```python
from build123d import *

# Parameters (mm, degrees)
F1_DEPTH        = 3.175
F2_R            = 6.35
F3_R            = 6.35
F5_DEPTH        = 34.7
F7_DEPTH        = 1.5875
F8_R            = 11.5
F9_DEPTH        = 215.1135
F11_D           = 4
F11_DEPTH       = 20
F11_START       = 1.5875
F11_CSINK_D     = 5
F11_CSINK_ANGLE = 90
F11_TIP         = 1.2017212381
F13_DEPTH       = 1.5875
F15_D           = 4
F15_DEPTH       = 20
F15_START       = 1.5875
F15_CSINK_D     = 5
F15_CSINK_ANGLE = 90
F15_TIP         = 1.2017212381
F17_D           = 4
F17_DEPTH       = 20
F17_TIP         = 1.2017212381
F20_D           = 4
F20_CSINK_D     = 8
F20_CSINK_ANGLE = 90


with BuildPart() as f1:
    # F0 (on Top) → F1 (new body)
    with BuildSketch(Plane.XY):
        Polygon((90.0875, 0), (0, 0), (0, -93.225), (216.7, -93.225), (216.7, -42.525), (126.6125, -42.525), (126.6125, 0), align=None)
    extrude(amount=F1_DEPTH)

    # F2
    f2_edges = [f1.edges().sort_by_distance(p)[0] for p in [
        (126.6125, -42.525, 1.5875),
    ]]
    fillet(f2_edges, radius=F2_R)

    # F3
    f3_edges = [f1.edges().sort_by_distance(p)[0] for p in [
        (216.7, -42.525, 1.5875),
        (216.7, -93.225, 1.5875),
        (0, -93.225, 1.5875),
        (0, 0, 1.5875),
    ]]
    fillet(f3_edges, radius=F3_R)

    # F4 (on face) → F5 (join)
    with BuildSketch(Plane.XY.offset(3.175)):
        with BuildLine():
            ThreePointArc((126.6125, -47.1735226281), (129.6754981272, -48.4422579939), (132.9625, -48.875))
            Line((132.9625, -48.875), (204, -48.875))
            ThreePointArc((204, -48.875), (208.4901280605, -50.7348719395), (210.35, -55.225))
            Line((210.35, -55.225), (210.35, -80.525))
            ThreePointArc((210.35, -80.525), (208.4901280605, -85.0151280605), (204, -86.875))
            Line((204, -86.875), (12.7, -86.875))
            ThreePointArc((12.7, -86.875), (8.2098719395, -85.0151280605), (6.35, -80.525))
            Line((6.35, -80.525), (6.35, -12.7))
            ThreePointArc((6.35, -12.7), (8.2098719395, -8.2098719395), (12.7, -6.35))
            Line((12.7, -6.35), (90.0875, -6.35))
            Line((90.0875, -6.35), (90.0875, 0))
            Line((90.0875, 0), (6.35, 0))
            ThreePointArc((6.35, 0), (1.8598719395, -1.8598719395), (0, -6.35))
            Line((0, -6.35), (0, -86.875))
            ThreePointArc((0, -86.875), (1.8598719395, -91.3651280605), (6.35, -93.225))
            Line((6.35, -93.225), (210.35, -93.225))
            ThreePointArc((210.35, -93.225), (214.8401280605, -91.3651280605), (216.7, -86.875))
            Line((216.7, -86.875), (216.7, -48.875))
            ThreePointArc((216.7, -48.875), (214.8401280605, -44.3848719395), (210.35, -42.525))
            Line((210.35, -42.525), (132.9625, -42.525))
            ThreePointArc((132.9625, -42.525), (128.4723719395, -40.6651280605), (126.6125, -36.175))
            Line((126.6125, -36.175), (126.6125, -47.1735226281))
        make_face()
    extrude(amount=F5_DEPTH)

    # F6 (on face) → F7 (cut)
    with BuildSketch(Plane.YZ.offset(216.7)):
        with BuildLine():
            ThreePointArc((-51.9375, 30.9375), (-53.1090728753, 33.7659271247), (-55.9375, 34.9375))
            Line((-55.9375, 34.9375), (-79.9375, 34.9375))
            ThreePointArc((-79.9375, 34.9375), (-82.7659271247, 33.7659271247), (-83.9375, 30.9375))
            Line((-83.9375, 30.9375), (-83.9375, 6.9375))
            ThreePointArc((-83.9375, 6.9375), (-82.7659271247, 4.1090728753), (-79.9375, 2.9375))
            Line((-79.9375, 2.9375), (-55.9375, 2.9375))
            ThreePointArc((-55.9375, 2.9375), (-53.1090728753, 4.1090728753), (-51.9375, 6.9375))
            Line((-51.9375, 6.9375), (-51.9375, 30.9375))
        make_face()
    extrude(amount=-F7_DEPTH, mode=Mode.SUBTRACT)

    # F8 (on face) → F9 (cut, through all)
    with BuildSketch(Plane.YZ.offset(215.1125)):
        with Locations((-67.9375, 18.9375)):
            Circle(F8_R)
    extrude(amount=-F9_DEPTH, mode=Mode.SUBTRACT)

    # F11
    # its depths count from where the whole tool has entered the part; down to there all is cleared
    with Locations(Plane.YZ.offset(216.7).offset(-F11_START)):
        with Locations((-79.251208499, 30.251208499), (-56.623791501, 30.251208499), (-56.623791501, 7.623791501), (-79.251208499, 7.623791501)):
            CounterSinkHole(F11_D / 2, F11_CSINK_D / 2, depth=F11_DEPTH, counter_sink_angle=F11_CSINK_ANGLE)
            with Locations((0, 0, -(F11_DEPTH + F11_TIP / 2))):  # 118° drill point
                Cone(0, F11_D / 2, F11_TIP, mode=Mode.SUBTRACT)

    # F12 (on face) → F13 (cut)
    with BuildSketch(Plane(origin=(0, 0, 0), x_dir=(0, -1, 0), z_dir=(-1, 0, 0))):
        with BuildLine():
            Line((79.9375, 34.9375), (55.9375, 34.9375))
            ThreePointArc((55.9375, 34.9375), (53.1090728753, 33.7659271247), (51.9375, 30.9375))
            Line((51.9375, 30.9375), (51.9375, 6.9375))
            ThreePointArc((51.9375, 6.9375), (53.1090728753, 4.1090728753), (55.9375, 2.9375))
            Line((55.9375, 2.9375), (79.9375, 2.9375))
            ThreePointArc((79.9375, 2.9375), (82.7659271247, 4.1090728753), (83.9375, 6.9375))
            Line((83.9375, 6.9375), (83.9375, 30.9375))
            ThreePointArc((83.9375, 30.9375), (82.7659271247, 33.7659271247), (79.9375, 34.9375))
        make_face()
    extrude(amount=-F13_DEPTH, mode=Mode.SUBTRACT)

    # F15
    # its depths count from where the whole tool has entered the part; down to there all is cleared
    with Locations(Plane(origin=(0, 0, 0), x_dir=(0, -1, 0), z_dir=(-1, 0, 0)).offset(-F15_START)):
        with Locations((56.623791501, 30.251208499), (56.623791501, 7.623791501), (79.251208499, 7.623791501), (79.251208499, 30.251208499)):
            CounterSinkHole(F15_D / 2, F15_CSINK_D / 2, depth=F15_DEPTH, counter_sink_angle=F15_CSINK_ANGLE)
            with Locations((0, 0, -(F15_DEPTH + F15_TIP / 2))):  # 118° drill point
                Cone(0, F15_D / 2, F15_TIP, mode=Mode.SUBTRACT)

    # F17
    with Locations(Plane.XY.offset(37.875)):
        with Locations((5, -5), (5, -88.225), (211.7, -88.225), (211.7, -47.525), (136.6125, -45.7), (83, -3.175), (108.35, -90.05)):
            Hole(F17_D / 2, depth=F17_DEPTH)
            with Locations((0, 0, -(F17_DEPTH + F17_TIP / 2))):  # 118° drill point
                Cone(0, F17_D / 2, F17_TIP, mode=Mode.SUBTRACT)

    # F20 (through all)
    with Locations(Plane(origin=(0, 0, 0), x_dir=(1, 0, 0), z_dir=(0, 0, -1))):
        with Locations((123.4375, 6.875), (123.4375, 42.875), (93.2625, 42.875), (93.2625, 6.875)):
            CounterSinkHole(F20_D / 2, F20_CSINK_D / 2, counter_sink_angle=F20_CSINK_ANGLE)


solid = f1.part
```
Geometry check sheet. Reference: the model listing, model coordinates, mm. A direction names the side the tool comes from. Round coordinates to 2 decimals unless told otherwise and drop trailing zeros. Write each loop counter-clockwise with the first axis right and the second up, starting at its lowest first coordinate (ties: lowest second). Pieces come first, ordered by that corner, then holes. Notation, with made-up numbers: (45, 56) -> (60, 56) arc R16 ccw to (60, 71) -> close; hole circle Ø1 at (42, 69). An arc over 180 degrees is marked (long way). Put each result on its own line as item: value.
1) Cross-section at D-D, the plane x = 150. Enter the section's corners in (y, z) (3 decimals), plus the area to 3 significant figures.
Recorded:
outline: (-93.225, 0) -> (-42.525, 0) -> (-42.525, 37.875) -> (-48.875, 37.875) -> (-48.875, 3.175) -> (-86.875, 3.175) -> (-86.875, 37.875) -> (-93.225, 37.875) -> close
area: 602 mm2
2) Depth check by flat-ended pin: P1, Ø5, axis at x = 123.44, y = -42.88, coming from the -Z side; P2, Ø4.5, axis at y = -79.25, z = 30.25, coming from the +X side; P3, Ø0.8, axis at x = 216, z = 22, coming from the -Y side. Enter the tip coordinate at first touch or a pass-through.
Recorded:
P1: stops at z = 1.49
P2: stops at x = 214.86
P3: stops at y = -90.45
3) Access from +Z, -Z, +X, -X, +Y, -Y to the whole of each face (thin tool, end or side, straight path). Record for faces 4 (the face through (8.26, -85.064, 20.282)), 5 (the face through (107, -93.225, 19)), 6 (the face through (0.783, -82.735, 4.078)).
Recorded:
face 4: +Z
face 5: +Z, -Z, +X, -X, -Y
face 6: -X
4) Release check for a two-part mould opening along X. For faces 1 (the face through (121.225, -7.572, 1.681)), 2 (the face through (212.43, -77.777, 31.603)), 3 (the face through (215, -79, 10)) record: pulls with the +X half, pulls with the -X half, needs draft (parallel to the pull), parting line crosses it, or undercut.
Recorded:
face 1: undercut
face 2: needs draft
face 3: pulls with the +X half
5) Cross-section at A-A, the plane x = 60.5. Enter the section's corners in (y, z) (3 decimals).
Recorded:
outline: (-93.225, 0) -> (0, 0) -> (0, 37.875) -> (-6.35, 37.875) -> (-6.35, 3.175) -> (-86.875, 3.175) -> (-86.875, 37.875) -> (-93.225, 37.875) -> close
6) Thickness scan on probe 1 along Y at (x, z) = (170.5, 6) (3 decimals); probe 2 along Y at (x, z) = (83, 26) (3 decimals); probe 3 along Y at (x, z) = (5, 29) (3 decimals). Record the ranges inside material, lowest first. Write a range as from..to.
Recorded:
probe 1: y = -93.225..-86.875, -48.875..-42.525
probe 2: y = -93.225..-86.875, -6.35..-5.175, -1.175..0
probe 3: y = -93.08..-90.225, -86.225..-80.811, -77.691..-73.505, -62.37..-58.184, -55.064..-7, -3..-0.145
7) Cross-section at B-B, the plane y = -72. Give the number of separate pieces and of enclosed holes in the cut face, plus the area to 3 significant figures.
Recorded:
separate pieces: 3
enclosed holes: 0
area: 822 mm2
